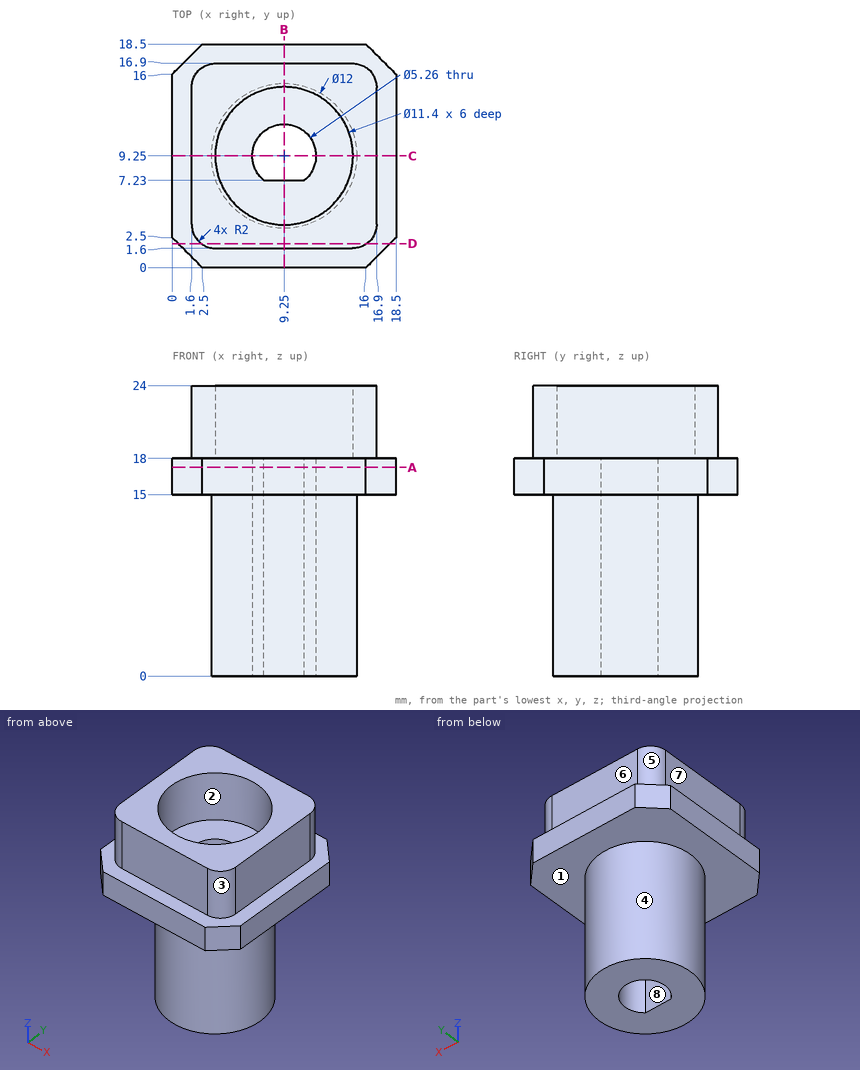
Input: dimensioned drawing with shaded views. Units: mm. Origin: part minimum x, y, z. A direction names the side the tool comes from. Give positions to 0.01 mm unless a question says otherwise; leave off trailing zeros. Write each loop counter-clockwise with the first axis right and the second up, starting at its lowest first coordinate (ties: lowest second). Pieces come first, ordered by that corner, then holes. Notation, with made-up numbers: (69.5, 7.25) - (73.5, 7.25) arc R23 cw to (73.5, 44.25) - close; hole circle Ø11 at (58.25, 11.25). An arc over 180 degrees is marked (long way). One line per item, written item: value. Start each with the question number.
Q1. Section query C-C, the plane y = 9.25. Return the cut outline in (x, z).
Q2. Section query A-A, the plane z = 17.25. Return the cut outline in (x, y).
Q3. Draft query along Y for the marked faces 1, 2 and 3. Return one class per face: +Y half, -Y half, draft (parallel to the pull), parting line (faces both ways), or undercut.
Q4. Material intervals for probe 1 along Y at (x, z) = (9.25, 19.8); probe 2 along X at (y, z) = (9.25, 6.75); probe 3 along Y at (x, z) = (9.25, 12), sorted ascending. Write a range as from..to.
Q5. Set-up query: the marked faces 4, 5, 6, 7 and 8. Return all of +Z, -Z, +X, -X, +Y, -Y with unobstructed straight access to the full face (end or side cutting, diameter ignored); none if empty.
Q6. Section query B-B, the plane x = 9.25. Return the cut outline in (y, z), then the cut area to 3 significant figures.
Q7. First-contact query: pin 1 Ø5 at (x, y) = (7.5, 4.5) entering from -Z; pin 2 Ø10.5 at (x, y) = (9.25, 9.25) entering from +Z; pin 3 Ø1 at (x, z) = (10.5, 6) entering from -Y; pin 4 Ø3.5 at (x, z) = (9.5, 12.5) entering from +Y. Flat tips, straight axial feed; report the tip coordinate or a pass-through.
Q8. Section query D-D, the plane y = 2. Return the cut outline in (x, z).
Answer:
1. outline: (0, 15) - (3.25, 15) - (3.25, 0) - (6.62, 0) - (6.62, 18) - (3.55, 18) - (3.55, 24) - (1.6, 24) - (1.6, 18) - (0, 18) - close; (11.88, 0) - (15.25, 0) - (15.25, 15) - (18.5, 15) - (18.5, 18) - (16.9, 18) - (16.9, 24) - (14.95, 24) - (14.95, 18) - (11.88, 18) - close
2. outline: (0, 2.5) - (2.5, 0) - (16, 0) - (18.5, 2.5) - (18.5, 16) - (16, 18.5) - (2.5, 18.5) - (0, 16) - close; hole (7.57, 7.23) - (10.93, 7.23) arc R2.63 ccw (long way) to start
3. face 1: draft
3. face 2: undercut
3. face 3: -Y half
4. probe 1: y = 1.6..3.55, 14.95..16.9
4. probe 2: x = 3.25..6.62, 11.88..15.25
4. probe 3: y = 3.25..7.23, 11.88..15.25
5. face 4: -Z
5. face 5: +Z, -X, +Y
5. face 6: +Z, +X, -X, +Y
5. face 7: +Z, -X, +Y, -Y
5. face 8: +Z, -Z
6. outline: (0, 15) - (3.25, 15) - (3.25, 0) - (7.23, 0) - (7.23, 18) - (3.55, 18) - (3.55, 24) - (1.6, 24) - (1.6, 18) - (0, 18) - close; (11.88, 0) - (15.25, 0) - (15.25, 15) - (18.5, 15) - (18.5, 18) - (16.9, 18) - (16.9, 24) - (14.95, 24) - (14.95, 18) - (11.88, 18) - close
6. area: 175 mm2
7. pin 1: stops at z = 0
7. pin 2: stops at z = 18
7. pin 3: stops at y = 3.3
7. pin 4: stops at y = 15.25
8. outline: (0.5, 15) - (18, 15) - (18, 18) - (16.1, 18) - (16.1, 24) - (2.4, 24) - (2.4, 18) - (0.5, 18) - close
